Read the model definition and answer for the solid it produces. Units are mm, in the model's axes. A direction names the side the tool comes from. Round coordinates to 2 decimals unless told otherwise and drop trailing zeros. Loops run counter-clockwise (first coordinate to the right, second up) from the corner with the lowest first, then second, coordinate; pieces in that order, holes last. Notation, with made-up numbers: (53, 32.5) - (89, 32.5) arc R20 ccw to (89, 57.5) - close; hole circle Ø6 at (80, -15.75). An arc over 180 degrees is marked (long way). Use one line per item in the form item = value. Start each with the question number.
```python
from build123d import *

# Parameters (mm, degrees)
F0_W     = 50
F0_H     = 46.1
F0_R     = 1.75
F1_DEPTH = 6
F2_W     = 50
F2_H     = 6.3
F3_DEPTH = 25


with BuildPart() as f1:
    # F0 (on Top) → F1 (new body)
    with BuildSketch(Plane.XY):
        Rectangle(F0_W, F0_H)
        with Locations((-19.95, 0)):
            Circle(F0_R, mode=Mode.SUBTRACT)
        with BuildLine():
            ThreePointArc((-13.4, 6.8), (-12.667767, 8.567767), (-10.9, 9.3))
            Line((-10.9, 9.3), (10.9, 9.3))
            ThreePointArc((10.9, 9.3), (12.667767, 8.567767), (13.4, 6.8))
            Line((13.4, 6.8), (13.4, -3.8))
            Line((13.4, -3.8), (8.30098, -9.3))
            Line((8.30098, -9.3), (-8.30098, -9.3))
            Line((-8.30098, -9.3), (-13.4, -3.8))
            Line((-13.4, -3.8), (-13.4, 6.8))
        make_face(mode=Mode.SUBTRACT)
        with Locations((19.95, 0)):
            Circle(F0_R, mode=Mode.SUBTRACT)
        with Locations((-19.95, 0)):
            Circle(F0_R)
        with Locations((19.95, 0)):
            Circle(F0_R)
    extrude(amount=F1_DEPTH)

    # F2 (on face) → F3 (join)
    with BuildSketch(Plane.XY):
        with Locations((0, 19.9)):
            Rectangle(F2_W, F2_H)
        with Locations((0, -19.9)):
            Rectangle(F2_W, F2_H)
    extrude(amount=-F3_DEPTH)


solid = f1.part
```
1) A cutting plane is placed at C-C on x = 19. Write down the section's boundary in (y, z).
2) Determine the mould class of faces 4 (the cylindrical face through (12.648, 8.587, 2.958)), 5 (the flat face through (0, 11, 6)), 6 (the flat face through (-25, 0, 1)) for opening direction X: +X half, -X half, draft (parallel to the pull), parting line (faces both ways), or undercut.
3) Straight lines are drawn through the part: line 1 (Y direction, x = 4.5, z = 5); line 2 (Y direction, x = -13, z = -19); line 3 (X direction, y = 7, z = 2). For each, find the intervals that lie inside material, in ascending order. Write a range as from..to.
4) A cutting plane is placed at B-B on z = 1.5. Write down the section's boundary in (x, y).
5) A cutting plane is placed at A-A on z = -10. Write down the section's boundary in (x, y), plus the area to 3 significant figures.
6) For faces 1 (the flat face through (0, 9.3, 3)), 2 (the flat face through (25, 0, 1)), 3 (the flat face through (0, -11, 0)), determine the directions among +Z, -Z, +X, -X, +Y, -Y from which every point of the face is accessible in a straight line to the end or side of a thin tool.
7) A cutting plane is placed at D-D on y = 2. Write down the section's boundary in (x, z), plus the area to 3 significant figures.
8) Flat-ended cylindrical pins translate along their axes: pin 1 (1 mm diameter, centred on y = -2, z = -1.5, fed in from +X); pin 2 (5 mm diameter, centred on x = 19, y = 7, fed in from -Z). Find the tip coordinate at first contact, or state that the pin passes through.
Checks:
q1.outline = (-23.05, -25) - (-16.75, -25) - (-16.75, 0) - (16.75, 0) - (16.75, -25) - (23.05, -25) - (23.05, 6) - (-23.05, 6) - close
q2.face_4 = undercut
q2.face_5 = draft
q2.face_6 = -X half
q3.line_1 = -23.05..-9.3, 9.3..23.05
q3.line_2 = -23.05..-16.75, 16.75..23.05
q3.line_3 = -25..-13.39, 13.39..25
q4.outline = (-25, -23.05) - (25, -23.05) - (25, 23.05) - (-25, 23.05) - close; hole (-13.4, -3.8) - (-8.3, -9.3) - (8.3, -9.3) - (13.4, -3.8) - (13.4, 6.8) arc R2.5 ccw to (10.9, 9.3) - (-10.9, 9.3) arc R2.5 ccw to (-13.4, 6.8) - close
q5.outline = (-25, -23.05) - (25, -23.05) - (25, -16.75) - (-25, -16.75) - close; (-25, 16.75) - (25, 16.75) - (25, 23.05) - (-25, 23.05) - close
q5.area = 630 mm²
q6.face_1 = +Z, -Z
q6.face_2 = +Z, -Z, +X, +Y, -Y
q6.face_3 = -Z, +X, -X
q7.outline = (-25, 0) - (-13.4, 0) - (-13.4, 6) - (-25, 6) - close; (13.4, 0) - (25, 0) - (25, 6) - (13.4, 6) - close
q7.area = 139 mm²
q8.pin_1 = through
q8.pin_2 = 0
